Autodesk Inventor part; units mm, degrees
ref_plane "YZ Plane" through (0, 0, 0) normal (1, 0, 0) x (0, 1, 0)
ref_plane "XZ Plane" through (0, 0, 0) normal (0, 1, 0) x (-1, 0, 0)
ref_plane "XY Plane" through (0, 0, 0) normal (0, 0, 1) x (1, 0, 0)
sketch "Sketch1" plane through (0, 0, 0) normal (0, 0, 1) x (1, 0, 0)
  line L0 (0, 0) -> (25.4, 0) construction
  line L1 (25.4, 0) -> (25.4, 76.2) construction
  line L2 (25.4, 76.2) -> (0, 76.2) construction
  line L3 (0, 76.2) -> (0, 0) construction
  line L4 (25.4, 0) -> (101.6, 0) construction
  line L5 (101.6, 0) -> (101.6, -25.4) construction
  line L6 (101.6, -25.4) -> (25.4, -25.4) construction
  line L7 (25.4, -25.4) -> (25.4, 0) construction
  line L8 (25.4, 0) -> (0, 0)
  line L9 (0, 25.4) -> (0, 0)
  line L10 (0, 25.4) -> (50.8, 25.4)
  line L11 (50.8, 25.4) -> (50.8, -25.4)
  line L12 (25.4, -25.4) -> (50.8, -25.4)
  line L13 (25.4, -25.4) -> (25.4, 0)
  point P0 (12.7, 6.35)
  point P1 (12.7, 19.05)
  point P2 (12.7, 12.7)
  point P3 (12.7, 0)
  point P4 (31.75, -12.7)
  point P5 (38.1, -12.7)
  point P6 (44.45, -12.7)
  point P7 (25.4, -12.7)
  dimension "d0" = 25.4
  dimension "d1" = 76.2
  dimension "d2" = 76.2
  dimension "d3" = 25.4
  dimension "d4" = 31.75
  dimension "d5" = 6.35
  dimension "d6" = 6.35
  dimension "d7" = 6.35
  dimension "d8" = 6.35
  dimension "d9" = 31.75
  dimension "d10" = 25.4
  dimension "d11" = 25.4
extrude "Extrusion1" add sketch "Sketch1" along normal blind 3.175
hole "Hole1" at (12.7, 6.35, 0) at (12.7, 19.05, 0) at (12.7, 12.7, 0) at (31.75, -12.7, 0) at (38.1, -12.7, 0) at (44.45, -12.7, 0) direction (0, 0, 1) diameter 5.1054 end through all
chamfer "Chamfer1" distance 19.05 angle 45 1 edges at (50.8, 25.4, 1.5875)
fillet "Fillet2" radius 6.35 2 edges at (31.75, 25.4, 1.5875) (50.8, 6.35, 1.5875)
equation "\"d10\" = d11"
properties part number "EL2-010" material "Aluminum 6061"
Part model, mm, in its own coordinate system. A direction names the side the tool comes from. Give positions to 0.01 mm unless a question says otherwise; leave off trailing zeros. Loops run counter-clockwise (first coordinate to the right, second up) from the corner with the lowest first, then second, coordinate; pieces in that order, holes last. Notation, with made-up numbers: (82.25, 47.25) -> (129.25, 47.25) arc R20 cw to (129.25, 71.25) -> close; hole circle Ø4 at (-1, 15.25). An arc over 180 degrees is marked (long way). Write each question's results on one line, items separated by ' | '. Start each with the question number.
Q1. Band-saw the part on A-A on y = 19.05. List the corners of the cut face in (x, z) (3 decimals), plus the area to 3 significant figures.
Q2. Band-saw the part on B-B on z = 2.1. List the corners of the cut face in (x, y).
Q3. Band-saw the part on C-C on x = 12.7. List the corners of the cut face in (y, z) (3 decimals).
Q4. Pull direction Y, two halves, no side cores. Call faces 3 (the face through (0, 13, 2)), 4 (the face through (41.92, -13.03, 1.61)), 5 (the face through (38, -25.4, 2)): +Y half, -Y half, draft (parallel to the pull), parting line (faces both ways), or undercut.
Q5. Which spindle directions (+Z, -Z, +X, -X, +Y, -Y) get a long thin tool onto all of the face, cutting with end or side? Do faces 1 (the face through (50.8, -11, 2)), 2 (the face through (25.4, -13, 2)). Say none if no direction does.
Q6. Band-saw the part on D-D on x = 43.5. List the corners of the cut face in (y, z) (3 decimals), plus the area to 3 significant figures.
Q7. Wall check: L1, parallel to X at y = -12.7, z = 1.95; L2, parallel to Y at x = 12.7, z = 2.4; L3, parallel to Y at x = 14, z = 1.2. Give the ranges that are in metal, low to high.
Q8. Pin check, flat tips, straight feed: P1, Ø4, axis at x = 44.45, y = -12.7, coming from the -Z side; P2, Ø1.6, axis at x = 17.5, z = 2, coming from the -Y side. Stop position of each tip, or through.
Results are:
1) outline: (0, 0) -> (10.147, 0) -> (10.147, 3.175) -> (0, 3.175) -> close; (15.253, 0) -> (38.1, 0) -> (38.1, 3.175) -> (15.253, 3.175) -> close | area: 105 mm²
2) outline: (0, 0) -> (25.4, 0) -> (25.4, -25.4) -> (50.8, -25.4) -> (50.8, 3.72) arc R6.35 ccw to (48.94, 8.21) -> (33.61, 23.54) arc R6.35 ccw to (29.12, 25.4) -> (0, 25.4) -> close; hole circle Ø5.11 at (12.7, 6.35); hole circle Ø5.11 at (12.7, 12.7); hole circle Ø5.11 at (12.7, 19.05); hole circle Ø5.11 at (31.75, -12.7); hole circle Ø5.11 at (38.1, -12.7); hole circle Ø5.11 at (44.45, -12.7)
3) outline: (0, 0) -> (3.797, 0) -> (3.797, 3.175) -> (0, 3.175) -> close; (8.903, 0) -> (10.147, 0) -> (10.147, 3.175) -> (8.903, 3.175) -> close; (15.253, 0) -> (16.497, 0) -> (16.497, 3.175) -> (15.253, 3.175) -> close; (21.603, 0) -> (25.4, 0) -> (25.4, 3.175) -> (21.603, 3.175) -> close
4) face 3: draft | face 4: undercut | face 5: -Y half
5) face 1: +Z, -Z, +X, +Y, -Y | face 2: +Z, -Z, -X, -Y
6) outline: (-25.4, 0) -> (-15.069, 0) -> (-15.069, 3.175) -> (-25.4, 3.175) -> close; (-10.331, 0) -> (13.65, 0) -> (13.65, 3.175) -> (-10.331, 3.175) -> close | area: 109 mm²
7) L1: x = 25.4 to 29.2, 34.3 to 35.55, 40.65 to 41.9, 47 to 50.8 | L2: y = 0 to 3.8, 8.9 to 10.15, 15.25 to 16.5, 21.6 to 25.4 | L3: y = 0 to 4.15, 8.55 to 10.5, 14.9 to 16.85, 21.25 to 25.4
8) P1: passes through | P2: stops at y = 0
